Verification items for the finished model (mm, model axes). Round coordinates to 2 decimals unless told otherwise and drop trailing zeros. Loops run counter-clockwise (first coordinate to the right, second up) from the corner with the lowest first, then second, coordinate; pieces in that order, holes last. Notation, with made-up numbers: M 53,55.5 L 61,55.5 A29 cw 61,79.5 Z; hole C 56,-27.75 d11. An arc over 180 degrees is marked long. One line per item, written item: value.
from build123d import *

# Parameters (mm, degrees)
SKETCH1_W           = 240
SKETCH1_H           = 157
BOSS_EXTRUDE1_DEPTH = 4
SKETCH2_R           = 3.5
CUT_EXTRUDE1_DEPTH  = 144.451211218
CUT_EXTRUDE2_DEPTH  = 4
SKETCH4_R           = 1.6
BOSS_EXTRUDE2_DEPTH = 4
SKETCH4_2_R         = 1.6
CUT_EXTRUDE3_DEPTH  = 4
SKETCH5_R           = 1.6
CUT_EXTRUDE5_DEPTH  = 4
BOSS_EXTRUDE4_DEPTH = 4
SKETCH6_R           = 7.5
CUT_EXTRUDE6_DEPTH  = 144.451211218
SKETCH7_W           = 65
SKETCH7_H           = 70
CUT_EXTRUDE7_DEPTH  = 144.451211218
SKETCH8_W           = 22.4
SKETCH8_H           = 29.4
CUT_EXTRUDE8_DEPTH  = 144.451211218


with BuildPart() as part:
    # Sketch1 → Boss-Extrude1 (new body)
    with BuildSketch(Plane.XY):
        Rectangle(SKETCH1_W, SKETCH1_H)
    extrude(amount=BOSS_EXTRUDE1_DEPTH)

    # Sketch2 → Cut-Extrude1 (cut, through all)
    with BuildSketch(Plane.XY.offset(4)):
        with Locations((-106.199999998, 68.5)):
            Circle(SKETCH2_R)
        with Locations((105.8, 68.5)):
            Circle(SKETCH2_R)
        with Locations((-0.199999998, -64.5)):
            Circle(SKETCH2_R)
    extrude(amount=-CUT_EXTRUDE1_DEPTH, mode=Mode.SUBTRACT)

    # Sketch3 → Cut-Extrude2 (cut)
    with BuildSketch(Plane(origin=(0, 0, 0), x_dir=(-1, 0, 0), z_dir=(0, 0, -1))):
        Polygon((-46, -74.5), (-116, -74.5), (-116, -14.5), (-91, -14.5), (-91, -10.5), (-71, -10.5), (-71, -14.5), (-46, -14.5), (-46, -34.5), (-42, -34.5), (-42, -54.5), (-46, -54.5), align=None)
    extrude(amount=-CUT_EXTRUDE2_DEPTH, mode=Mode.SUBTRACT)

    # Sketch4 → Boss-Extrude2 (add)
    with BuildSketch(Plane.XY.offset(4)):
        with Locations((44, -24.5)):
            Circle(SKETCH4_R)
        with BuildLine():
            Line((46, -21.035898385), (46, -27.964101615))
            ThreePointArc((46, -27.964101615), (48, -24.5), (46, -21.035898385))
        make_face()
    boss_extrude2 = extrude(amount=-BOSS_EXTRUDE2_DEPTH)

    # Sketch4<2> → Cut-Extrude3 (cut)
    with BuildSketch(Plane.XY.offset(4)):
        with Locations((44, -24.5)):
            Circle(SKETCH4_2_R)
    cut_extrude3 = extrude(amount=-CUT_EXTRUDE3_DEPTH, mode=Mode.SUBTRACT)

    # Mirror1: Boss-Extrude2, Cut-Extrude3 across plane
    add(boss_extrude2.mirror(Plane(origin=(0, -44.5, 0), x_dir=(0, 0, 1), z_dir=(0, -1, 0))))
    add(cut_extrude3.mirror(Plane(origin=(0, -44.5, 0), x_dir=(0, 0, 1), z_dir=(0, -1, 0))), mode=Mode.SUBTRACT)

    # Sketch5 → Cut-Extrude5 (cut)
    with BuildSketch(Plane.XY.offset(4)):
        with Locations((58.5, -12.5)):
            Circle(SKETCH5_R)
    cut_extrude5 = extrude(amount=-CUT_EXTRUDE5_DEPTH, mode=Mode.SUBTRACT)

    # Sketch5<5> → Boss-Extrude4 (add)
    with BuildSketch(Plane.XY.offset(4)):
        with BuildLine():
            Line((61.964101615, -14.5), (55.035898385, -14.5))
            ThreePointArc((55.035898385, -14.5), (58.5, -16.5), (61.964101615, -14.5))
        make_face()
    boss_extrude4 = extrude(amount=-BOSS_EXTRUDE4_DEPTH)

    # Mirror3: Cut-Extrude5, Boss-Extrude4 across plane
    add(cut_extrude5.mirror(Plane(origin=(81, 0, 0), x_dir=(0, 0, 1), z_dir=(1, 0, 0))), mode=Mode.SUBTRACT)
    add(boss_extrude4.mirror(Plane(origin=(81, 0, 0), x_dir=(0, 0, 1), z_dir=(1, 0, 0))))

    # Sketch6 → Cut-Extrude6 (cut, through all)
    with BuildSketch(Plane(origin=(0, 0, 0), x_dir=(-1, 0, 0), z_dir=(0, 0, -1))):
        with Locations((60, 1.5)):
            Circle(SKETCH6_R)
    extrude(amount=-CUT_EXTRUDE6_DEPTH, mode=Mode.SUBTRACT)

    # Sketch7 → Cut-Extrude7 (cut, through all)
    with BuildSketch(Plane.XY.offset(4)):
        with Locations((0, -19.5)):
            Rectangle(SKETCH7_W, SKETCH7_H)
    extrude(amount=-CUT_EXTRUDE7_DEPTH, mode=Mode.SUBTRACT)

    # Sketch8 → Cut-Extrude8 (cut, through all)
    with BuildSketch(Plane(origin=(0, 0, 0), x_dir=(-1, 0, 0), z_dir=(0, 0, -1))):
        with Locations((97.5, -52.5)):
            Rectangle(SKETCH8_W, SKETCH8_H)
    extrude(amount=-CUT_EXTRUDE8_DEPTH, mode=Mode.SUBTRACT)


solid = part.part
(1) Sectioned sample at C-C on x = -60. Enter the section's corners in (y, z), and give its area (3 significant figures).
Completed:
outline: M -78.5,0 L -6,0 L -6,4 L -78.5,4 Z; M 9,0 L 78.5,0 L 78.5,4 L 9,4 Z
area: 568 mm^2
(2) Mould release check, pull along Z, two halves, no side actions. Record for faces 1 (the face through (-28, 19, 4)), 2 (the face through (102.303, 68.654, 2.028)), 3 (the face through (-28, 19, 0)): +Z half, -Z half, draft (parallel to the pull), parting line (faces both ways), or undercut.
Completed:
face 1: +Z half
face 2: draft
face 3: -Z half
(3) Thickness scan on L1, parallel to Y at x = 0, z = 3.1; L2, parallel to Y at x = 44, z = 1.85; L3, parallel to X at y = -29.5, z = 3.45. Record the ranges inside material, lowest first. Write a range as from..to.
Completed:
L1: y = -78.5..-67.99, -61.01..-54.5, 15.5..78.5
L2: y = -78.5..-66.1, -62.9..-54.5, -34.5..-26.1, -22.9..78.5
L3: x = -120..-32.5, 32.5..46, 116..120
(4) Depth check by flat-ended pin: pin 1 Ø3.5 at (x, y) = (44, -24.5) entering from +Z. Enter the tip coordinate at first touch or a pass-through.
Completed:
pin 1: stops at z = 4
(5) Sectioned sample at A-A on x = 85.5. Enter the section's corners in (y, z), and give its area (3 significant figures).
Completed:
outline: M -78.5,0 L -74.5,0 L -74.5,4 L -78.5,4 Z; M -10.5,0 L 78.5,0 L 78.5,4 L -10.5,4 Z
area: 372 mm^2
(6) Sectioned sample at D-D on z = 2.65. Count the separate pieces of the cut face and the enclosed holes in it, and give its area (3 significant figures).
Completed:
separate pieces: 1
enclosed holes: 11
area: 27,800 mm^2
(7) Sectioned sample at B-B on x = -106.2. Enter the section's corners in (y, z).
Completed:
outline: M -78.5,0 L -67.2,0 L -67.2,4 L -78.5,4 Z; M -37.8,0 L 65,0 L 65,4 L -37.8,4 Z; M 72,0 L 78.5,0 L 78.5,4 L 72,4 Z
